from build123d import *

# Parameters (mm, degrees)
EXTRUDE_1_DEPTH     = 4
FILLET_1_R          = 4
FILLET_2_R          = 10
SKETCH_8_R          = 4.9
SKETCH_8_R_2        = 1.65
SKETCH_8_R_3        = 2
CUT_EXTRUDE_1_DEPTH = 5


with BuildPart() as part:
    # 草图1 → 凸台-拉伸1 (new body)
    with BuildSketch(Plane(origin=(0, 0, 0), x_dir=(1, 0, 0), z_dir=(0, 1, 0))):
        Polygon((60, 100), (-60, 100), (-100, 60), (-100, 35), (-75, 35), (-75, -35), (-100, -35), (-100, -60), (-60, -100), (60, -100), (100, -60), (100, -35), (75, -35), (75, 35), (100, 35), (100, 60), align=None)
    extrude(amount=EXTRUDE_1_DEPTH)

    # 圆角1
    fillet_1_edges = [part.edges().sort_by_distance(p)[0] for p in [
        (100, 2, 35),
        (-100, 2, 35),
        (-75, 2, 35),
        (-75, 2, -35),
        (-100, 2, -35),
        (100, 2, -35),
        (75, 2, -35),
        (75, 2, 35),
    ]]
    fillet(fillet_1_edges, radius=FILLET_1_R)

    # 圆角2
    fillet_2_edges = [part.edges().sort_by_distance(p)[0] for p in [
        (100, 2, 60),
        (60, 2, 100),
        (-60, 2, 100),
        (-100, 2, 60),
        (-100, 2, -60),
        (-60, 2, -100),
        (60, 2, -100),
        (100, 2, -60),
    ]]
    fillet(fillet_2_edges, radius=FILLET_2_R)

    # 草图8 → 切除-拉伸1 (cut, through all)
    with BuildSketch(Plane(origin=(0, 4, 0), x_dir=(1, 0, 0), z_dir=(0, 1, 0))):
        with Locations((-60.5, 0)):
            Circle(SKETCH_8_R)
        with Locations((-67.5, 8)):
            Circle(SKETCH_8_R_2)
        with Locations((-53.5, 8)):
            Circle(SKETCH_8_R_2)
        with Locations((-53.5, -8)):
            Circle(SKETCH_8_R_2)
        with Locations((-67.5, -8)):
            Circle(SKETCH_8_R_2)
        with Locations((53.5, -8)):
            Circle(SKETCH_8_R_2)
        with Locations((67.5, -8)):
            Circle(SKETCH_8_R_2)
        with Locations((60.5, 0)):
            Circle(SKETCH_8_R)
        with Locations((53.5, 8)):
            Circle(SKETCH_8_R_2)
        with Locations((67.5, 8)):
            Circle(SKETCH_8_R_2)
        with Locations((-17.5, 80)):
            Circle(SKETCH_8_R_3)
        with Locations((17.5, 80)):
            Circle(SKETCH_8_R_3)
        with Locations((17.5, -80)):
            Circle(SKETCH_8_R_3)
        with Locations((-17.5, -80)):
            Circle(SKETCH_8_R_3)
        Circle(SKETCH_8_R_3)
        with Locations((-78.939339828, -69.746951673)):
            Circle(SKETCH_8_R_3)
        with Locations((-69.746951673, -78.939339828)):
            Circle(SKETCH_8_R_3)
        with Locations((69.746951673, -78.939339828)):
            Circle(SKETCH_8_R_3)
        with Locations((78.939339828, -69.746951673)):
            Circle(SKETCH_8_R_3)
    extrude(amount=-CUT_EXTRUDE_1_DEPTH, mode=Mode.SUBTRACT)


solid = part.part
The listing builds one solid part. Answer for the finished solid, in the listing's coordinates (mm). Round coordinates to 2 decimals unless told otherwise and drop trailing zeros. Order: outer loops, then holes, each group sorted by start corner. A loop starts at its lowest first (then second) coordinate and runs counter-clockwise, first axis right, second up. Notation, with made-up numbers: M 55,62.5 L 102,62.5 A17 ccw 102,87.5 Z; hole C -26,57 d3. An arc over 180 degrees is marked long. Answer in a Markdown table with one row per item. Add a question column.
1) The part is cut by section B-B on x = -60.5. Determine the outline of the cut face in (y, z).
2) Determine the mould class of faces 1 (the face through (65.174, 2.028, -1.472)), 2 (the face through (80, 2, -80)), 3 (the face through (-80, 2, -80)), 4 (the face through (-55.826, 2.028, -1.472)) for opening direction X: pulls with the +X half, pulls with the -X half, needs draft (parallel to the pull), parting line crosses it, or undercut.
3) The part is cut by section A-A on x = 58.5. Determine the outline of the cut face in (y, z).
4) The part is cut by section C-C on y = 1.65. Count the separate pieces of the cut face and the enclosed holes in it, plus the area to 3 significant figures.
5) Flat-ended cylindrical pins translate along their axes: pin 1 Ø8 at (x, z) = (60.5, 0) entering from -Y; pin 2 Ø2 at (x, y) = (-89, 2) entering from +Z; pin 3 Ø2 at (y, z) = (2.5, -10) entering from +X; pin 4 Ø1.2 at (x, y) = (-86.5, 2) entering from -Z. Find the tip coordinate at first contact, or state that the pin passes through.
6) Consider line 1 along Z through (x, y) = (-17.5, 3); line 2 along X through (y, z) = (2.75, -8); line 3 along Z through (x, y) = (-53.5, 2.1). Determine where each line is inside the solid, lowest interval first. Write a range as from..to.
Findings below:
| question | item | result |
|---|---|---|
| 1 | outline | M 0,-98.86 L 4,-98.86 L 4,-4.9 L 0,-4.9 Z; M 0,4.9 L 4,4.9 L 4,98.86 L 0,98.86 Z |
| 2 | face 1 | undercut |
| 2 | face 2 | pulls with the +X half |
| 2 | face 3 | pulls with the -X half |
| 2 | face 4 | undercut |
| 3 | outline | M 0,-99.64 L 4,-99.64 L 4,-4.47 L 0,-4.47 Z; M 0,4.47 L 4,4.47 L 4,99.64 L 0,99.64 Z |
| 4 | separate pieces | 1 |
| 4 | enclosed holes | 19 |
| 4 | area | 33,000 mm² |
| 5 | pin 1 | passes through |
| 5 | pin 2 | stops at z = 72 |
| 5 | pin 3 | stops at x = 75 |
| 5 | pin 4 | stops at z = -74.1 |
| 6 | line 1 | z = -100..-82, -78..78, 82..100 |
| 6 | line 2 | x = -75..-69.15, -65.85..-55.15, -51.85..51.85, 55.15..65.85, 69.15..75 |
| 6 | line 3 | z = -100..-9.65, -6.35..6.35, 9.65..100 |
